For this review, take the finished solid that the model builds, in its own axes (mm). Round coordinates to 2 decimals unless told otherwise and drop trailing zeros. Loops run counter-clockwise (first coordinate to the right, second up) from the corner with the lowest first, then second, coordinate; pieces in that order, holes last.
1) Take a section at C-C (x = -22.5). State the section outline as (y, z) points, then the cut area to 3 significant figures.
2) Wall thickness on L1, parallel to Y at x = -22.5, z = 0.3; L2, parallel to Y at x = -21.5, z = 0.1; L3, parallel to Y at x = -39.5, z = 0.9: over which ranges is each line inside the solid? List them lowest first.
3) Take a section at B-B (y = 3.25). State the section outline as (x, z) points.
4) Take a section at D-D (y = -1). State the section outline as (x, z) points, then the cut area to 3 significant figures.
5) Insertion check: pin 1 (4 mm diameter, centred on x = -37.68, y = 1.1, fed in from -Z). The pin has a flat end and moves straight along its axis. Give the tip position at first contact, or say it passes through.
6) Take a section at A-A (z = 0.2). State the section outline as (x, y) points, then the cut area to 3 significant figures.
Autodesk Inventor part; units mm, degrees
ref_plane "YZ Plane" through (0, 0, 0) normal (1, 0, 0) x (0, 1, 0)
ref_plane "XZ Plane" through (0, 0, 0) normal (0, 1, 0) x (-1, 0, 0)
ref_plane "XY Plane" through (0, 0, 0) normal (0, 0, 1) x (1, 0, 0)
sketch "Sketch1" plane through (0, 0, 0) normal (0, 0, 1) x (1, 0, 0)
  line L0 (-12.5, -2.5) -> (-12.5, 2.5)
  line L1 (-12.5, 2.5) -> (-17.5, 2.5)
  line L2 (-17.5, 2.5) -> (-17.5, 7.5)
  line L3 (-32.5, 7.5) -> (-17.5, 7.5)
  arc A0 (-32.5, 7.5) -> (-12.5, -2.5) centre (-12.5, 22.5) ccw
  circle A1 centre (-22.5, 4) radius 1.75
  circle A2 centre (-37.6776, 1.0985) radius 1.75
  line L4 (-22.5, 4) -> (-37.6776, 1.0985)
  line L5 (-22.5, 4) -> (-21.7788, 0.2278)
  line L6 (-22.5, 4) -> (-21.9367, 1.0534)
  line L7 (-37.6776, 1.0985) -> (-37.1143, -1.8482)
  line L8 (-21.9367, 1.0534) -> (-37.1143, -1.8482)
  line L9 (-22.5, 4) -> (-19.5534, 4.5633)
  line L10 (-21.9367, 1.0534) -> (-18.99, 1.6167)
  line L11 (-18.99, 1.6167) -> (-19.5534, 4.5633)
  line L12 (-37.6776, 1.0985) -> (-38.2409, 4.0451)
  line L13 (-23.0633, 6.9466) -> (-38.2409, 4.0451)
  line L14 (-23.0633, 6.9466) -> (-20.1167, 7.51)
  line L15 (-20.1167, 7.51) -> (-19.5534, 4.5633)
  line L16 (-37.1143, -1.8482) -> (-40.0609, -2.4115)
  line L17 (-40.0609, -2.4115) -> (-41.1875, 3.4818)
  line L18 (-41.1875, 3.4818) -> (-38.2409, 4.0451)
  line L19 (-18.99, 1.6167) -> (-40.0609, -2.4115)
  line L20 (-40.0609, -2.4115) -> (-41.1875, 3.4818)
  line L21 (-41.1875, 3.4818) -> (-20.1167, 7.51)
  point P0 (0, 0)
  dimension "d0" = 3.5
  dimension "d1" = 3.5
  dimension "d2" = 90
  dimension "d3" = 3
  dimension "d4" = 3
  dimension "d5" = 180
  dimension "d6" = 3
extrude "Extrusion1" add sketch "Sketch1" along normal blind 1 contours L8 L7 A2 L4 A0 | A0 L4 A1 L5 L8 | L4 A2 L12 L13 A0 | A0 L13 L14 L3 L15 L9 A1 L4 | L5 A1 L9 L11 L10 | L16 L17 L18 L12 A2 L7 | L4 L5 A1 | L4 L12 A2 | A2 L7 L4 | L5 L9 A1 | A2 L12 L7 | L3 L14 L15
sketch "Sketch2" plane through (0, 0, 1) normal (0, 0, 1) x (1, 0, 0)
  arc A0 (-20.7811, 4.3286) -> (-24.2189, 3.6714) centre (-22.5, 4) ccw
  line L0 (-68.111, -8.1624) -> (-72.0972, 25.6031)
  line L1 (-29.38, -3.59) -> (-68.111, -8.1624)
  line L2 (-33.3662, 30.1755) -> (-29.38, -3.59)
  line L3 (-72.0972, 25.6031) -> (-33.3662, 30.1755)
  line L4 (-24.2189, 3.6714) -> (-20.7811, 4.3286)
  circle A1 centre (-22.5, 4) radius 1.75
  line L5 (-37.6776, 1.0985) -> (-35.9587, 1.4271)
  circle A2 centre (-37.6776, 1.0985) radius 1.75
  point P0 (0, 0)
extrude "Extrusion2" cut sketch "Sketch2" against normal blind 1 contours L4 A0 | A1 L4 | A2
fillet "Fillet1" radius 1 4 edges at (-40.0609, -2.4115, 0.5) (-41.1875, 3.4818, 0.5) (-18.99, 1.6167, 0.5) (-20.1167, 7.51, 0.5)
properties part number "LeverArm"
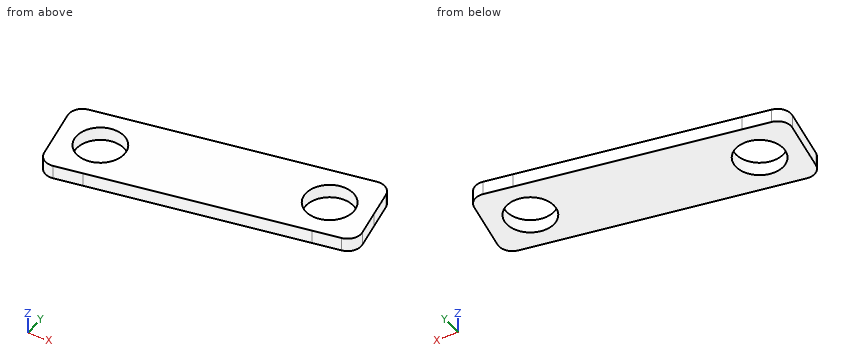
Response:
1. outline: (0.95, 0) - (2.25, 0) - (2.25, 1) - (0.95, 1) - close; (5.75, 0) - (7.05, 0) - (7.05, 1) - (5.75, 1) - close
1. area: 2.61 mm2
2. L1: y = 0.95 to 2.25, 5.75 to 7.05
2. L2: y = 1.14 to 2.56, 5.44 to 7.25
2. L3: y = -2.21 to 3.8
3. outline: (-40.84, 0) - (-24.08, 0) - (-24.08, 1) - (-40.84, 1) - close; (-20.92, 0) - (-19.3, 0) - (-19.3, 1) - (-20.92, 1) - close
4. outline: (-40.33, 0) - (-32.68, 0) - (-32.68, 1) - (-40.33, 1) - close
4. area: 7.65 mm2
5. pin 1: stops at z = 0
6. outline: (-41, 2.5) - (-40.25, -1.43) arc R1 ccw to (-39.08, -2.22) - (-37.11, -1.85) - (-21.94, 1.05) - (-19.97, 1.43) arc R1 ccw to (-19.18, 2.6) - (-19.55, 4.56) - (-19.93, 6.53) arc R1 ccw to (-21.1, 7.32) - (-23.06, 6.95) - (-38.24, 4.05) - (-40.21, 3.67) arc R1 ccw to start; hole circle Ø3.5 at (-37.68, 1.1); hole circle Ø3.5 at (-22.5, 4)
6. area: 109 mm2
